from build123d import *

# Parameters (mm, degrees)
F0_W           = 31
F0_H           = 42
F0_R           = 1.15
F0_W_2         = 21
F0_H_2         = 32
F1_DEPTH       = 6.5
F2_W           = 31
F2_H           = 42
F2_R           = 1.15
F2_W_2         = 21
F2_H_2         = 32
F3_DEPTH       = 4
F4_W           = 13
F4_H           = 5
F4_W_2         = 7
F5_DEPTH       = 6
F6_R           = 2
F8_D           = 2.9
F8_CBORE_D     = 5.5
F8_CBORE_DEPTH = 2.5


with BuildPart() as f1:
    # F0 (on Top) → F1 (new body)
    with BuildSketch(Plane.XY):
        Rectangle(F0_W, F0_H)
        with Locations((-13, -18.5)):
            Circle(F0_R, mode=Mode.SUBTRACT)
        with Locations((13, -18.5)):
            Circle(F0_R, mode=Mode.SUBTRACT)
        with Locations((-13, 18.5)):
            Circle(F0_R, mode=Mode.SUBTRACT)
        Rectangle(F0_W_2, F0_H_2, mode=Mode.SUBTRACT)
        with Locations((13, 18.5)):
            Circle(F0_R, mode=Mode.SUBTRACT)
    extrude(amount=F1_DEPTH)

    # F2 (on face) → F3 (join)
    with BuildSketch(Plane(origin=(0, 0, 0), x_dir=(1, 0, 0), z_dir=(0, 0, -1))):
        Rectangle(F2_W, F2_H)
        with Locations((-13, -18.5)):
            Circle(F2_R, mode=Mode.SUBTRACT)
        with Locations((13, -18.5)):
            Circle(F2_R, mode=Mode.SUBTRACT)
        with Locations((-13, 18.5)):
            Circle(F2_R, mode=Mode.SUBTRACT)
        Rectangle(F2_W_2, F2_H_2, mode=Mode.SUBTRACT)
        with Locations((13, 18.5)):
            Circle(F2_R, mode=Mode.SUBTRACT)
        with Locations((-13, 18.5)):
            Circle(F2_R)
        with Locations((13, 18.5)):
            Circle(F2_R)
        with Locations((-13, -18.5)):
            Circle(F2_R)
        Rectangle(F2_W_2, F2_H_2)
        with Locations((13, -18.5)):
            Circle(F2_R)
    extrude(amount=F3_DEPTH)

    # F4 (on face) → F5 (cut)
    with BuildSketch(Plane.XY.offset(6.5)):
        with Locations((0, -18.5)):
            Rectangle(F4_W, F4_H)
        with Locations((0, 18.5)):
            Rectangle(F4_W_2, F4_H)
    extrude(amount=-F5_DEPTH, mode=Mode.SUBTRACT)

    # F6
    f6_edges = [f1.edges().sort_by_distance(p)[0] for p in [
        (-15.5, 21, 1.25),
        (15.5, 21, 1.25),
        (15.5, -21, 1.25),
        (-15.5, -21, 1.25),
    ]]
    fillet(f6_edges, radius=F6_R)

    # F8 (through all)
    with Locations(Plane.XY):
        with Locations((0, 10), (0, -10)):
            CounterBoreHole(F8_D / 2, F8_CBORE_D / 2, F8_CBORE_DEPTH)


solid = f1.part
Verification items for the finished model (mm, model axes). A direction names the side the tool comes from. Give positions to 0.01 mm unless a question says otherwise; leave off trailing zeros. Order: outer loops, then holes, each group sorted by start corner. A loop starts at its lowest first (then second) coordinate and runs counter-clockwise, first axis right, second up. Notation, with made-up numbers: M -18.75,15.25 L -6.75,15.25 A20 cw -6.75,30.25 Z; hole C 17,-22 d1. An arc over 180 degrees is marked long. Use one line per item in the form item = value. Start each with the question number.
Q1. Section check B-B (y = -10). Enter the section's corners in (x, z), then the cut area to 3 significant figures.
Q2. Go/stop test with flat-tipped pins: pin 1 Ø3.5 at (x, y) = (13, -18.5) entering from +Z; pin 2 Ø6 at (x, y) = (-1, -11) entering from +Z; pin 3 Ø1.6 at (x, y) = (1.5, 11) entering from +Z; pin 4 Ø2.5 at (x, y) = (0.5, -19.5) entering from +Z. Record where each tip stops, or that it passes through.
Q3. Mould release check, pull along X, two halves, no side actions. Record for faces 1 (the cylindrical face through (-14.93, 20.4, 1.18)), 2 (the cylindrical face through (-13.249, 17.377, 3.204)), 3 (the flat face through (12, 0, 6.5)): +X half, -X half, draft (parallel to the pull), parting line (faces both ways), or undercut.
Q4. Access from +Z, -Z, +X, -X, +Y, -Y to the whole of each face (thin tool, end or side, straight path). Record for faces 4 (the flat face through (0, 19, 0.5)), 5 (the flat face through (-6.5, -19, 4)), 6 (the flat face through (-10.5, 0, 3)), 7 (the flat face through (0, 21, 0)).
Q5. Section check C-C (x = 6). Enter the section's corners in (y, z).
Q6. Scan lines: line 1 along Y through (x, z) = (0, -3.2); line 2 along Y through (x, z) = (0, -1.15); line 3 along Z through (x, y) = (-1, 5). Record each from-to range of solid material in increasing order. Write a range as [from, to].
Q7. Section check D-D (y = -18.5). Enter the section's corners in (x, z), then the cut area to 3 significant figures.
Q8. Section check A-A (z = 3.5). Enter the section's corners in (x, y).
Evaluation:
q1.outline = M -15.5,-4 L -1.45,-4 L -1.45,-2.5 L -2.75,-2.5 L -2.75,0 L -10.5,0 L -10.5,6.5 L -15.5,6.5 Z; M 1.45,-4 L 15.5,-4 L 15.5,6.5 L 10.5,6.5 L 10.5,0 L 2.75,0 L 2.75,-2.5 L 1.45,-2.5 Z
q1.area = 171 mm2
q2.pin_1 = 6.5
q2.pin_2 = 0
q2.pin_3 = -2.5
q2.pin_4 = 0.5
q3.face_1 = -X half
q3.face_2 = undercut
q3.face_3 = draft
q4.face_4 = +Z, +Y, -Y
q4.face_5 = +Z, -Y
q4.face_6 = +Z
q4.face_7 = +Z, -Z, +X, -X, +Y
q5.outline = M -21,-4 L 21,-4 L 21,6.5 L 16,6.5 L 16,0 L -16,0 L -16,0.5 L -21,0.5 Z
q6.line_1 = [-21, -11.45], [-8.55, 8.55], [11.45, 21]
q6.line_2 = [-21, -12.75], [-7.25, 7.25], [12.75, 21]
q6.line_3 = [-4, 0]
q7.outline = M -15.5,-4 L 15.5,-4 L 15.5,6.5 L 14.15,6.5 L 14.15,0 L 11.85,0 L 11.85,6.5 L 6.5,6.5 L 6.5,0.5 L -6.5,0.5 L -6.5,6.5 L -11.85,6.5 L -11.85,0 L -14.15,0 L -14.15,6.5 L -15.5,6.5 Z
q7.area = 218 mm2
q8.outline = M -15.5,-19 A2 ccw -13.5,-21 L -6.5,-21 L -6.5,-16 L -10.5,-16 L -10.5,16 L -3.5,16 L -3.5,21 L -13.5,21 A2 ccw -15.5,19 Z; M 3.5,16 L 10.5,16 L 10.5,-16 L 6.5,-16 L 6.5,-21 L 13.5,-21 A2 ccw 15.5,-19 L 15.5,19 A2 ccw 13.5,21 L 3.5,21 Z; hole C -13,-18.5 d2.3; hole C -13,18.5 d2.3; hole C 13,-18.5 d2.3; hole C 13,18.5 d2.3
